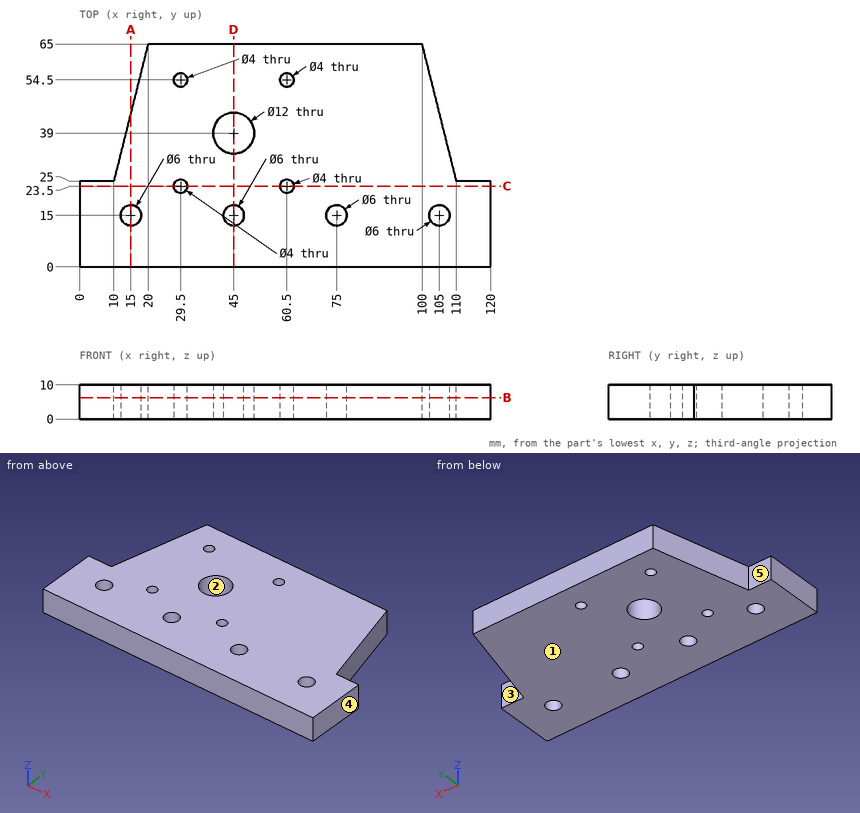
Answer from the drawing. Dimensions are ordinates in mm from the lowest x, y and z of the part. A direction names the side the tool comes from. Round coordinates to 2 decimals unless told otherwise and drop trailing zeros. Loops run counter-clockwise (first coordinate to the right, second up) from the corner with the lowest first, then second, coordinate; pieces in that order, holes last. Notation, with made-up numbers: (-40, 13.25) - (-33, 13.25) arc R22 cw to (-33, 21.25) - close; hole circle Ø7 at (38, 41). An arc over 180 degrees is marked (long way). One line per item, written item: value.
Q1. Find section C-C on y = 23.5. Give the vertices of the cut face in (x, z).
Check values:
outline: (0, 0) - (27.5, 0) - (27.5, 10) - (0, 10) - close; (31.5, 0) - (58.5, 0) - (58.5, 10) - (31.5, 10) - close; (62.5, 0) - (120, 0) - (120, 10) - (62.5, 10) - close
Q2. The mould has two halves that part along Y. Classify the marked faces 1, 2 and 3: +Y half, -Y half, draft (parallel to the pull), parting line (faces both ways), or undercut.
Check values:
face 1: draft
face 2: undercut
face 3: +Y half
Q3. Find section B-B on z = 6.25. State how many separate pieces and enclosed holes the cut face has, and give its area (3 significant figures).
Check values:
separate pieces: 1
enclosed holes: 9
area: 6,320 mm2
Q4. Each of these flat-tipped pins is pushed along its axis until it touches: pin 1 Ø5.5 at (x, y) = (105, 15) entering from -Z; pin 2 Ø3 at (x, z) = (4.5, 3) entering from +Y; pin 3 Ø1 at (y, z) = (50.5, 4.5) entering from -X; pin 4 Ø6 at (y, z) = (52.5, 6) entering from -X (3 decimals). Where does it stop, or does it pass through?
Check values:
pin 1: through
pin 2: y = 25
pin 3: x = 16.25
pin 4: x = 16.125
Q5. Find section A-A on x = 15. Give the vertices of the cut face in (y, z).
Check values:
outline: (0, 0) - (12, 0) - (12, 10) - (0, 10) - close; (18, 0) - (45, 0) - (45, 10) - (18, 10) - close
Q6. Straight lines are drawn through the part: probe 1 along Y at (x, z) = (29.5, 7.25); probe 2 along X at (y, z) = (15, 1.75); probe 3 along X at (y, z) = (54.5, 3.75) (3 decimals). For each, find the intervals that lie inside material, in ascending order.
Check values:
probe 1: 0 to 21.5, 25.5 to 52.5, 56.5 to 65
probe 2: 0 to 12, 18 to 42, 48 to 72, 78 to 102, 108 to 120
probe 3: 17.375 to 27.5, 31.5 to 58.5, 62.5 to 102.625
Q7. Find section D-D on x = 45. Give the vertices of the cut face in (y, z).
Check values:
outline: (0, 0) - (12, 0) - (12, 10) - (0, 10) - close; (18, 0) - (33, 0) - (33, 10) - (18, 10) - close; (45, 0) - (65, 0) - (65, 10) - (45, 10) - close
Q8. For the marked faces 4 and 5, determine the directions among +Z, -Z, +X, -X, +Y, -Y from which every point of the face is accessible in a straight line to the end or side of a thin tool.
Check values:
face 4: +Z, -Z, +X, +Y, -Y
face 5: +Z, -Z, -X, +Y
